from build123d import *

# Parameters (mm, degrees)
BOSS_EXTRUDE1_DEPTH = 38.1
SKETCH2_R           = 8.7503
BOSS_EXTRUDE2_DEPTH = 38.1
BOSS_EXTRUDE6_DEPTH = 11.572281197
BOSS_EXTRUDE9_DEPTH = 15.24


with BuildPart() as part:
    # Sketch1 → Boss-Extrude1 (new body)
    with BuildSketch(Plane.XY):
        Polygon((0, 0), (142.319474343, 0), (142.319474343, 67.883016851), (85.129737171, 67.883016851), (85.129737171, 53.144138708), (110.529737171, 53.144138708), (110.529737171, 40.190138708), (31.789737171, 40.190138708), (31.789737171, 53.144138708), (57.189737171, 53.144138708), (57.189737171, 67.883016851), (0, 67.883016851), align=None)
    extrude(amount=BOSS_EXTRUDE1_DEPTH)



with BuildPart() as body_2:
    # Sketch2 → Boss-Extrude2 (new body)
    with BuildSketch(Plane.XY.offset(38.1)):
        with Locations((71.120000025, -35.559977798)):
            Circle(SKETCH2_R)
    extrude(amount=-BOSS_EXTRUDE2_DEPTH)


with BuildPart() as part_1:
    add(part.part)

    add(body_2.part)  # Boss-Extrude6 merges body 2
    # Sketch8 → Boss-Extrude6 (add)
    with BuildSketch(Plane.XY.offset(38.1)):
        with BuildLine():
            Line((63.59200581, -40.020589099), (63.59200581, 0))
            Line((63.59200581, 0), (78.647994227, 0))
            Line((78.647994227, 0), (78.647994227, -40.020589121))
            ThreePointArc((78.647994227, -40.020589121), (71.120000012, -44.310277798), (63.59200581, -40.020589099))
        make_face()
    extrude(amount=-BOSS_EXTRUDE6_DEPTH)

    # Sketch11 → Boss-Extrude9 (add)
    with BuildSketch(Plane(origin=(78.647994227, 0, 0), x_dir=(0, 0, -1), z_dir=(1, 0, 0))):
        Polygon((-26.527718803, -31.099366474), (0, 0), (-13.263859401, 0), (-26.527718803, -15.549683237), align=None)
    extrude(amount=-BOSS_EXTRUDE9_DEPTH)


solid = part_1.part
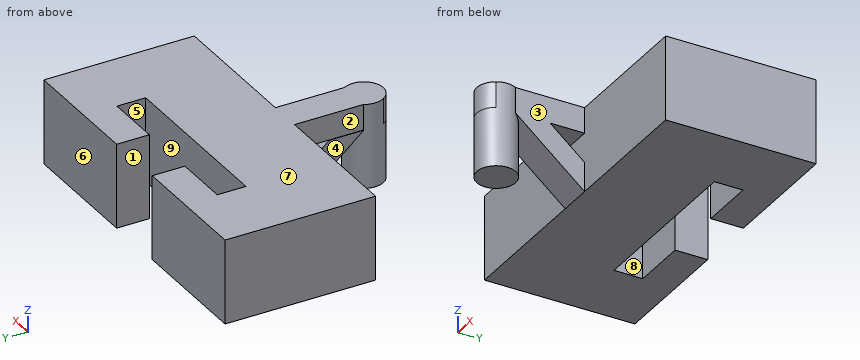
The model under review builds one solid part; all positions refer to its coordinate system, in mm. Face numbers are marked on the shaded views. A direction names the side the tool comes from. Give positions to 0.01 mm unless a question says otherwise; leave off trailing zeros. Order: outer loops, then holes, each group sorted by start corner. A loop starts at its lowest first (then second) coordinate and runs counter-clockwise, first axis right, second up. Notation, with made-up numbers: (41.25, 60) -> (64.25, 60) arc R29 ccw to (64.25, 96) -> close; hole circle Ø11 at (15, -17). An arc over 180 degrees is marked (long way). Write item = value, one per line. Start each with the question number.
(1) For pin 1 Ø2 at (x, z) = (64, 14) entering from +Y; pin 2 Ø1.5 at (x, y) = (115, 27) entering from -Z; pin 3 Ø1.5 at (y, z) = (-29, 16) entering from -X; pin 4 Ø9.5 at (y, z) = (-21.5, 32.5) entering from -X, all flat-tipped, find the tip position at first contact; note any pin that passes through.
(2) Take a section at A-A (x = 95.5). Write out the cut boundary in (y, z), plus the area to 3 significant figures.
(3) Take a section at C-C (x = 71.12). Write out the cut boundary in (y, z).
(4) For L1, parallel to X at y = 56.5, z = 15; L2, parallel to X at y = 50.5, z = 29.5; L3, parallel to Y at x = 100, z = 31, list the stretches that pass through material, from the lowest coordinate up. Write a range as from..to.
(5) Draft analysis for pull direction Y (two halves, no side actions). For the marked faces 6, 7, 8 and 9, state which applies: +Y half, -Y half, draft (parallel to the pull), parting line (faces both ways), or undercut.
(6) Tool access review of the marked faces 1, 2, 3, 4 and 5: name each direction out of +Z, -Z, +X, -X, +Y, -Y from which nothing blocks a thin tool from reaching the whole face with its end or side.
(7) Take a section at B-B (z = 23). Write out the cut boundary in (x, y), plus the area to 3 significant figures.
Returned:
q1.pin_1 = 40.19
q1.pin_2 = 0
q1.pin_3 = 64.58
q1.pin_4 = 63.59
q2.outline = (0, 0) -> (40.19, 0) -> (40.19, 38.1) -> (0, 38.1) -> close; (53.14, 0) -> (67.88, 0) -> (67.88, 38.1) -> (53.14, 38.1) -> close
q2.area = 2,090 mm²
q3.outline = (-44.31, 0) -> (-26.81, 0) -> (-26.81, 22.87) -> (0, 0) -> (40.19, 0) -> (40.19, 38.1) -> (-44.31, 38.1) -> close; hole (-15.55, 26.53) -> (0, 13.26) -> (0, 26.53) -> close
q4.L1 = 0..57.19, 85.13..142.32
q4.L2 = 0..31.79, 110.53..142.32
q4.L3 = 0..40.19, 53.14..67.88
q5.face_6 = +Y half
q5.face_7 = draft
q5.face_8 = undercut
q5.face_9 = undercut
q6.face_1 = +Z, -Z, +Y
q6.face_2 = +Z, -X
q6.face_3 = +Z, -Z, +X
q6.face_4 = +Z, -Z, -X
q6.face_5 = +Z, -Z
q7.outline = (0, 0) -> (142.32, 0) -> (142.32, 67.88) -> (85.13, 67.88) -> (85.13, 53.14) -> (110.53, 53.14) -> (110.53, 40.19) -> (31.79, 40.19) -> (31.79, 53.14) -> (57.19, 53.14) -> (57.19, 67.88) -> (0, 67.88) -> close; (63.41, -26.96) -> (69.49, -26.96) arc R8.75 ccw (long way) to (72.75, -26.96) -> (78.65, -26.96) -> (78.65, -11.41) -> (63.41, -11.41) -> close
q7.area = 8,710 mm²
